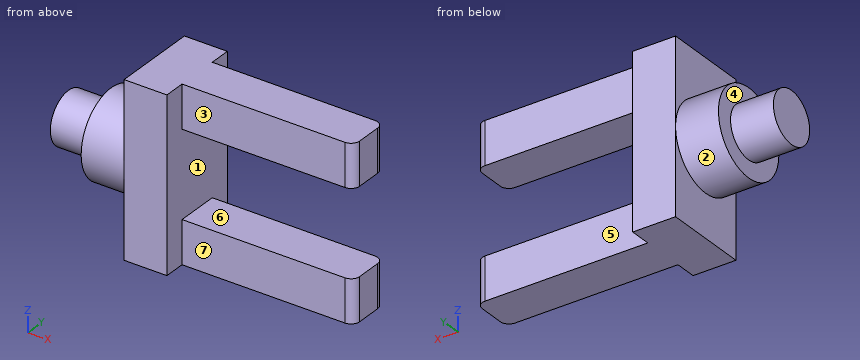
from build123d import *

# Parameters (mm, degrees)
SKETCH1_R           = 10
BOSS_EXTRUDE1_DEPTH = 20
SKETCH2_OUTSIDE_W   = 28.928
SKETCH2_OUTSIDE_H   = 28.928
SKETCH2_OUTSIDE_R   = 6
CUT_EXTRUDE1_DEPTH  = 10
SKETCH4_W           = 40
SKETCH4_H           = 20
BOSS_EXTRUDE2_DEPTH = 10
SKETCH6_W           = 10
SKETCH6_H           = 10
BOSS_EXTRUDE3_DEPTH = 40
SKETCH7_W           = 10
SKETCH7_H           = 10
BOSS_EXTRUDE4_DEPTH = 40
FILLET1_R           = 2


with BuildPart() as part:
    # Sketch1 → Boss-Extrude1 (new body)
    with BuildSketch(Plane(origin=(0, 0, 0), x_dir=(0, 0, -1), z_dir=(1, 0, 0))):
        Circle(SKETCH1_R)
    extrude(amount=BOSS_EXTRUDE1_DEPTH)

    # Sketch2 outside → Cut-Extrude1 (cut)
    with BuildSketch(Plane.ZY):
        Rectangle(SKETCH2_OUTSIDE_W, SKETCH2_OUTSIDE_H)
        Circle(SKETCH2_OUTSIDE_R, mode=Mode.SUBTRACT)
    extrude(amount=-CUT_EXTRUDE1_DEPTH, mode=Mode.SUBTRACT)

    # Sketch4 → Boss-Extrude2 (add)
    with BuildSketch(Plane(origin=(20, 0, 0), x_dir=(0, 0, -1), z_dir=(1, 0, 0))):
        Rectangle(SKETCH4_W, SKETCH4_H)
    extrude(amount=BOSS_EXTRUDE2_DEPTH)

    # Sketch6 → Boss-Extrude3 (add)
    with BuildSketch(Plane(origin=(30, 0, 0), x_dir=(0, 0, -1), z_dir=(1, 0, 0))):
        with Locations((-15, 0)):
            Rectangle(SKETCH6_W, SKETCH6_H)
    extrude(amount=BOSS_EXTRUDE3_DEPTH)

    # Sketch7 → Boss-Extrude4 (add)
    with BuildSketch(Plane(origin=(30, 0, 0), x_dir=(0, 0, -1), z_dir=(1, 0, 0))):
        with Locations((15, 0)):
            Rectangle(SKETCH7_W, SKETCH7_H)
    extrude(amount=BOSS_EXTRUDE4_DEPTH)

    # Fillet1
    fillet1_edges = [part.edges().sort_by_distance(p)[0] for p in [
        (70, -5, -15),
        (70, 5, -15),
        (70, -5, 15),
        (70, 5, 15),
    ]]
    fillet(fillet1_edges, radius=FILLET1_R)


solid = part.part
Read the model definition and answer for the solid it produces. Units are mm, in the model's axes. Face numbers are marked on the shaded views. A direction names the side the tool comes from. Coordinates: 2 decimals unless noted, no trailing zeros. Loops run counter-clockwise (first coordinate to the right, second up) from the corner with the lowest first, then second, coordinate; pieces in that order, holes last.
Q1. The mould has two halves that part along Z. Classify the marked faces 1, 2 and 3: +Z half, -Z half, draft (parallel to the pull), parting line (faces both ways), or undercut.
Q2. Consider probe 1 along Z at (x, y) = (60, 0.25); probe 2 along Y at (x, z) = (62, -10.5); probe 3 along X at (y, z) = (-6.5, -3). Determine where each line is inside the solid, lowest interval first.
Q3. The part is cut by section B-B on y = 0. Write down the section's boundary in (x, z).
Q4. The part is cut by section A-A on x = 53. Write down the section's boundary in (y, z).
Q5. The part is cut by section C-C on z = -2. Write down the section's boundary in (x, y).
Q6. The part is cut by section D-D on x = 16. Write down the section's boundary in (y, z).
Q7. Which of the six approach directions +Z, -Z, +X, -X, +Y, -Y give full straight-line access (tool end or side, diameter ignored) to the marked faces 4, 5, 6 and 7?
Q8. Each of these flat-tipped pins is pushed along its axis until it touches: pin 1 Ø6 at (x, z) = (46, 9.5) entering from +Y; pin 2 Ø5 at (x, z) = (40.5, 15.5) entering from -Y; pin 3 Ø4 at (x, y) = (12.5, 6.5) entering from -Z. Where does it stop, or does it pass through?
Results below:
1. face 1: undercut
1. face 2: parting line
1. face 3: draft
2. probe 1: z = -20 to -10, 10 to 20
2. probe 2: y = -5 to 5
2. probe 3: x = 10 to 30
3. outline: (0, -6) - (10, -6) - (10, -10) - (20, -10) - (20, -20) - (70, -20) - (70, -10) - (30, -10) - (30, 10) - (70, 10) - (70, 20) - (20, 20) - (20, 10) - (10, 10) - (10, 6) - (0, 6) - close
4. outline: (-5, -20) - (5, -20) - (5, -10) - (-5, -10) - close; (-5, 10) - (5, 10) - (5, 20) - (-5, 20) - close
5. outline: (0, -5.66) - (10, -5.66) - (10, -9.8) - (20, -9.8) - (20, -10) - (30, -10) - (30, 10) - (20, 10) - (20, 9.8) - (10, 9.8) - (10, 5.66) - (0, 5.66) - close
6. outline: circle Ø20 at (0, 0)
7. face 4: -X
7. face 5: +Z, -Z, +X, +Y
7. face 6: +X, +Y, -Y
7. face 7: +Z, -Z, +X, -Y
8. pin 1: stops at y = 5
8. pin 2: stops at y = -5
8. pin 3: stops at z = -8.93
